```python
from build123d import *

# Parameters (mm, degrees)
SKETCH_1_R      = 2
EXTRUDE_1_DEPTH = 1.5


with BuildPart() as part:
    # 草图1 → 凸台-拉伸1 (new, symmetric)
    with BuildSketch(Plane.XY):
        with BuildLine():
            Line((-34.285, 24.845), (34.285, 24.845))
            ThreePointArc((34.285, 24.845), (37.488193719, 23.518193719), (38.815, 20.315))
            Line((38.815, 20.315), (38.815, -20.315))
            ThreePointArc((38.815, -20.315), (37.488193719, -23.518193719), (34.285, -24.845))
            Line((34.285, -24.845), (-34.285, -24.845))
            ThreePointArc((-34.285, -24.845), (-37.488193719, -23.518193719), (-38.815, -20.315))
            Line((-38.815, -20.315), (-38.815, 20.315))
            ThreePointArc((-38.815, 20.315), (-37.488193719, 23.518193719), (-34.285, 24.845))
        make_face()
        with Locations((34.29, 20.32)):
            Circle(SKETCH_1_R, mode=Mode.SUBTRACT)
        with Locations((34.29, -20.32)):
            Circle(SKETCH_1_R, mode=Mode.SUBTRACT)
        with Locations((-34.29, 20.32)):
            Circle(SKETCH_1_R, mode=Mode.SUBTRACT)
        with Locations((-34.285, -20.315)):
            Circle(SKETCH_1_R, mode=Mode.SUBTRACT)
    extrude(amount=EXTRUDE_1_DEPTH, both=True)


solid = part.part
```
Check sheet for the modelled part. Datum: model origin and axes. Units: mm. Give positions to 0.01 mm unless a question says otherwise; leave off trailing zeros. Write each loop counter-clockwise with the first axis right and the second up, starting at its lowest first coordinate (ties: lowest second). Pieces come first, ordered by that corner, then holes.
Item 1: Gauge pin test, flat end, axial feed: pin 1 (5 mm diameter, centred on x = -34.285, y = -20.315, fed in from +Z). Record the tip position at first contact, or that the pin passes through.
Item 2: Draft check along X on faces 1 (the face through (-32.443, 19.554, -0.021)), 2 (the face through (0, 24.845, 0)), 3 (the face through (-37.523, 23.483, 0.021)), 4 (the face through (-34.719, -22.267, -0.021)). Enter one of: released by +X, released by -X, zero draft, split by the parting line, or undercut.
Item 3: Cross-section at A-A (z = 0.25). Enter the section's corners in (x, y) (3 decimals), and give its area (3 significant figures).
Item 4: Scan lines: L1, parallel to Y at x = -34.29, z = -0.65 (3 decimals); L2, parallel to X at y = 19, z = -1.2 (3 decimals); L3, parallel to X at y = 19.5, z = 1.45 (3 decimals). Record each from-to range of solid material in increasing order.
Report:
1. pin 1: stops at z = 1.5
2. face 1: undercut
2. face 2: zero draft
2. face 3: released by -X
2. face 4: undercut
3. outline: (-38.815, -20.315) arc R4.53 ccw to (-34.285, -24.845) - (34.285, -24.845) arc R4.53 ccw to (38.815, -20.315) - (38.815, 20.315) arc R4.53 ccw to (34.285, 24.845) - (-34.285, 24.845) arc R4.53 ccw to (-38.815, 20.315) - close; hole circle Ø4 at (-34.29, 20.32); hole circle Ø4 at (-34.285, -20.315); hole circle Ø4 at (34.29, -20.32); hole circle Ø4 at (34.29, 20.32)
3. area: 3,790 mm2
4. L1: y = -24.845 to -22.315, -18.315 to 18.32, 22.32 to 24.845
4. L2: x = -38.815 to -35.793, -32.787 to 32.787, 35.793 to 38.815
4. L3: x = -38.815 to -36.114, -32.466 to 32.466, 36.114 to 38.815
